Autodesk Inventor part; units mm, degrees
ref_plane "YZ Plane" through (0, 0, 0) normal (1, 0, 0) x (0, 1, 0)
ref_plane "XZ Plane" through (0, 0, 0) normal (0, 1, 0) x (-1, 0, 0)
ref_plane "XY Plane" through (0, 0, 0) normal (0, 0, 1) x (1, 0, 0)
sketch "Sketch1" plane through (0, 0, 0) normal (0, 0, 1) x (1, 0, 0)
  line L0 (-75, -40) -> (75, -40)
  line L1 (75, -40) -> (75, 40)
  line L2 (75, 40) -> (-75, 40)
  line L3 (-75, 40) -> (-75, -40)
  line L4 (-75, -40) -> (75, 40) construction
  line L5 (75, -40) -> (-75, 40) construction
  point P0 (0, 0)
  dimension "d0" = 80
  dimension "d1" = 150
extrude "Extrusion1" add sketch "Sketch1" along normal blind 5
sketch "Sketch2" plane through (0, 0, 5) normal (0, 0, 1) x (1, 0, 0)
  line L0 (29, -14.15) -> (51, -14.15) construction
  line L1 (51, -14.15) -> (51, 14.15) construction
  line L2 (51, 14.15) -> (29, 14.15) construction
  line L3 (29, 14.15) -> (29, -14.15) construction
  line L4 (29, -14.15) -> (51, 14.15) construction
  line L5 (51, -14.15) -> (29, 14.15) construction
  line L6 (-65, -16.5) -> (-15, -16.5) construction
  line L7 (-15, -16.5) -> (-15, 16.5) construction
  line L8 (-15, 16.5) -> (-65, 16.5) construction
  line L9 (-65, 16.5) -> (-65, -16.5) construction
  line L10 (-65, -16.5) -> (-15, 16.5) construction
  line L11 (-15, -16.5) -> (-65, 16.5) construction
  point P0 (0, 0)
  point P1 (40, 0)
  point P2 (-40, 0)
  point P3 (-40, 0)
  point P4 (40, 0)
  point P5 (29, 0)
  dimension "d4" = 50
  dimension "d5" = 33
  dimension "d6" = 40
  dimension "d7" = 28.3
  dimension "d8" = 22
  dimension "d9" = 40
hole "Hole1" at (51, 14.15, 5) at (51, -14.15, 5) at (29, 0, 5) at (-15, -16.5, 5) at (-15, 16.5, 5) at (-65, 16.5, 5) at (-65, -16.5, 5) direction (0, 0, -1) diameter 3.4 depth 8 tip angle 118
sketch "Sketch3" plane through (0, 0, 5) normal (0, 0, 1) x (1, 0, 0)
  line L0 (-50, 38) -> (50, 38) construction
  line L1 (50, 38) -> (50, 33) construction
  line L2 (50, 33) -> (-50, 33) construction
  line L3 (-50, 33) -> (-50, 38) construction
  line L4 (-50, 38) -> (50, 33) construction
  line L5 (50, 38) -> (-50, 33) construction
  line L6 (-50, -33) -> (50, -33) construction
  line L7 (50, -33) -> (50, -38) construction
  line L8 (50, -38) -> (-50, -38) construction
  line L9 (-50, -38) -> (-50, -33) construction
  line L10 (-50, -33) -> (50, -38) construction
  line L11 (50, -33) -> (-50, -38) construction
  line L12 (75, 40) -> (-75, 40)
  line L13 (-75, -40) -> (75, -40)
  line L14 (-50, 38) -> (-10, 38)
  line L15 (-10, 38) -> (-10, 33)
  line L16 (-10, 33) -> (-50, 33)
  line L17 (-50, 33) -> (-50, 38)
  line L18 (50, 38) -> (10, 38)
  line L19 (10, 38) -> (10, 33)
  line L20 (10, 33) -> (50, 33)
  line L21 (50, 33) -> (50, 38)
  line L22 (50, -33) -> (10, -33)
  line L23 (10, -33) -> (10, -38)
  line L24 (10, -38) -> (50, -38)
  line L25 (50, -38) -> (50, -33)
  line L26 (-50, -33) -> (-10, -33)
  line L27 (-10, -33) -> (-10, -38)
  line L28 (-10, -38) -> (-50, -38)
  line L29 (-50, -38) -> (-50, -33)
  point P0 (0, 0)
  point P1 (0, 35.5)
  point P2 (0, -35.5)
  point P3 (0, 35.5)
  point P4 (0, -35.5)
  dimension "d17" = 5
  dimension "d18" = 5
  dimension "d19" = 2
  dimension "d20" = 2
  dimension "d21" = 100
  dimension "d22" = 20
  dimension "d23" = 10
extrude "Extrusion2" cut sketch "Sketch3" against normal blind 5
fillet "Fillet1" radius 4 4 edges at (75, 40, 2.5) (75, -40, 2.5) (-75, -40, 2.5) (-75, 40, 2.5)
sketch "Sketch4" plane through (0, 0, 5) normal (0, 0, 1) x (1, 0, 0)
  line L0 (-10, -38) -> (-50, -38)
  line L1 (-50, 38) -> (-10, 38)
  point P0 (0, 0)
  point P1 (0, 35.5)
  point P2 (0, -35.5)
  dimension "d27" = 2.5
  dimension "d28" = 2.5
hole "Hole2" at (0, 35.5, 5) at (0, -35.5, 5) direction (0, 0, -1) diameter 3.4 depth 8 tip angle 118
properties part number "Interrupter_Bottom" material "Polycarbonate, Clear"
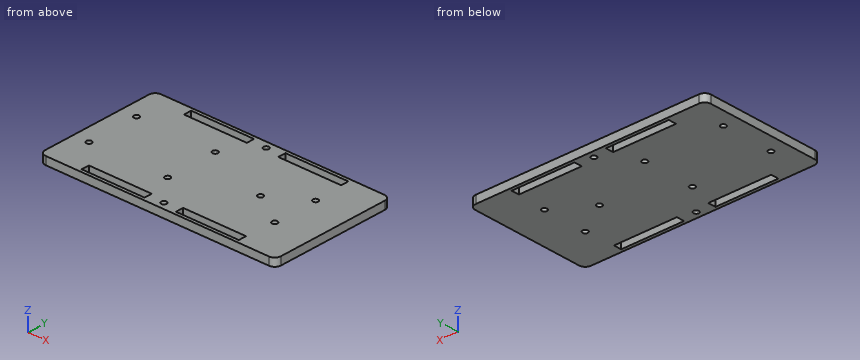
Input: part model. Units: mm. Frame: model coordinates. Coordinates: 2 decimals unless noted, no trailing zeros. Order: outer loops, then holes, each group sorted by start corner. A loop starts at its lowest first (then second) coordinate and runs counter-clockwise, first axis right, second up. Notation, with made-up numbers: M -40,-1.75 L 1,-1.75 A19 cw 1,26.25 Z; hole C 27,80.5 d10. An arc over 180 degrees is marked long. Answer as CSV lines item,"result".
1. Section B-B (x = -15). Return the cut outline in (y, z), then the cut area to 3 significant figures.
Reported:
outline,"M -40,0 L -38,0 L -38,5 L -40,5 Z; M -33,0 L -18.2,0 L -18.2,5 L -33,5 Z; M -14.8,0 L 14.8,0 L 14.8,5 L -14.8,5 Z; M 18.2,0 L 33,0 L 33,5 L 18.2,5 Z; M 38,0 L 40,0 L 40,5 L 38,5 Z"
area,"316 mm2"
2. Section D-D (x = 14). Return the cut outline in (y, z).
Reported:
outline,"M -40,0 L -38,0 L -38,5 L -40,5 Z; M -33,0 L 33,0 L 33,5 L -33,5 Z; M 38,0 L 40,0 L 40,5 L 38,5 Z"
3. Section C-C (z = 3). State how many separate pieces and enclosed holes the cut face has, then the cut area to 3 significant figures.
Reported:
separate pieces,"1"
enclosed holes,"13"
area,"11,100 mm2"
4. Section A-A (x = -65). Return the cut outline in (y, z), then the cut area to 3 significant figures.
Reported:
outline,"M -40,0 L -18.2,0 L -18.2,5 L -40,5 Z; M -14.8,0 L 14.8,0 L 14.8,5 L -14.8,5 Z; M 18.2,0 L 40,0 L 40,5 L 18.2,5 Z"
area,"366 mm2"
5. Material intervals for line 1 (Y direction, x = 51, z = 3.45); line 2 (Y direction, x = -27.5, z = 2); line 3 (X direction, y = 16.5, z = 1.25), sorted ascending. Write a range as from..to.
Reported:
line 1,"-40..-15.85, -12.45..12.45, 15.85..40"
line 2,"-40..-38, -33..33, 38..40"
line 3,"-75..-66.7, -63.3..-16.7, -13.3..75"
6. First-contact query: P1, Ø6, axis at x = 51, y = 3.5, coming from the -Z side; P2, Ø3, axis at x = -65, y = -16.5, coming from the -Z side. Flat tips, straight axial feed; report the tip coordinate or a pass-through.
Reported:
P1,"z = 0"
P2,"through"
